The drawing under review shows one solid part. Ordinate dimensions are in mm from its lowest x, y, z. A direction names the side the tool comes from. Give positions to 0.01 mm unless a question says otherwise; leave off trailing zeros. Loops run counter-clockwise (first coordinate to the right, second up) from the corner with the lowest first, then second, coordinate; pieces in that order, holes last. Notation, with made-up numbers: (-19.75, -15) - (17.25, -15) arc R24 cw to (17.25, 22) - close; hole circle Ø4 at (41.25, -36.75). An arc over 180 degrees is marked (long way). Put each result on its own line as item: value. Start each with the question number.
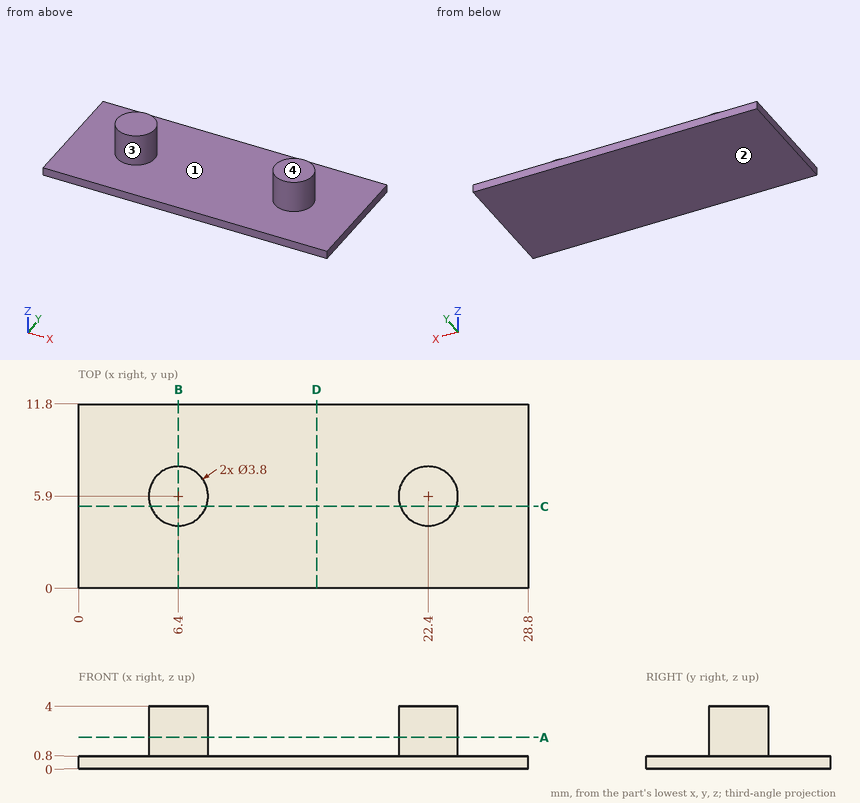
Item 1: Consider section C-C (y = 5.25). State the section outline as (x, z) points, plus the area to 3 significant figures.
Item 2: Machinability: for the marked faces 1 and 2, which of the approach directions +Z, -Z, +X, -X, +Y, -Y give a long, thin tool a straight path to every point of the face, cutting with its end or side? Answer none if there is none.
Item 3: Consider section A-A (z = 2). State the section outline as (x, y) points, plus the area to 3 significant figures.
Item 4: Mouldability with a two-part tool opening along X and no side actions: class the marked faces 3 and 4 as pulls with the +X half, pulls with the -X half, needs draft (parallel to the pull), parting line crosses it, or undercut.
Item 5: For L1, parallel to Z at x = 21, y = 10.75; L2, parallel to X at y = 5.75, z = 3.5; L3, parallel to X at y = 4.25, z = 2.45, list the stretches that pass through material, from the lowest coordinate up. Write a range as from..to.
Item 6: Consider section D-D (x = 15.25). State the section outline as (y, z) points, plus the area to 3 significant figures.
Item 7: For P1, Ø1.5, axis at x = 4.5, y = 8.5, coming from the +Z side; P2, Ø1, axis at y = 7.5, z = 2.5, coming from the +X side, all flat-tipped, find the tip position at first contact; note any pin that passes through.
Item 8: Consider section B-B (x = 6.4). State the section outline as (y, z) points, plus the area to 3 significant figures.
Geometry says:
1. outline: (0, 0) - (28.8, 0) - (28.8, 0.8) - (24.19, 0.8) - (24.19, 4) - (20.61, 4) - (20.61, 0.8) - (8.19, 0.8) - (8.19, 4) - (4.61, 4) - (4.61, 0.8) - (0, 0.8) - close
1. area: 45.9 mm2
2. face 1: +Z
2. face 2: -Z, +X, -X, +Y, -Y
3. outline: circle Ø3.8 at (6.4, 5.9); circle Ø3.8 at (22.4, 5.9)
3. area: 22.7 mm2
4. face 3: undercut
4. face 4: needs draft
5. L1: z = 0..0.8
5. L2: x = 4.51..8.29, 20.51..24.29
5. L3: x = 5.46..7.34, 21.46..23.34
6. outline: (0, 0) - (11.8, 0) - (11.8, 0.8) - (0, 0.8) - close
6. area: 9.44 mm2
7. P1: stops at z = 0.8
7. P2: stops at x = 23.95
8. outline: (0, 0) - (11.8, 0) - (11.8, 0.8) - (7.8, 0.8) - (7.8, 4) - (4, 4) - (4, 0.8) - (0, 0.8) - close
8. area: 21.6 mm2
